Work out the finished part from the listing and answer in its coordinate system (mm). Face numbers are marked on the shaded views. A direction names the side the tool comes from. Round coordinates to 2 decimals unless told otherwise and drop trailing zeros. One line per item, written item: value.
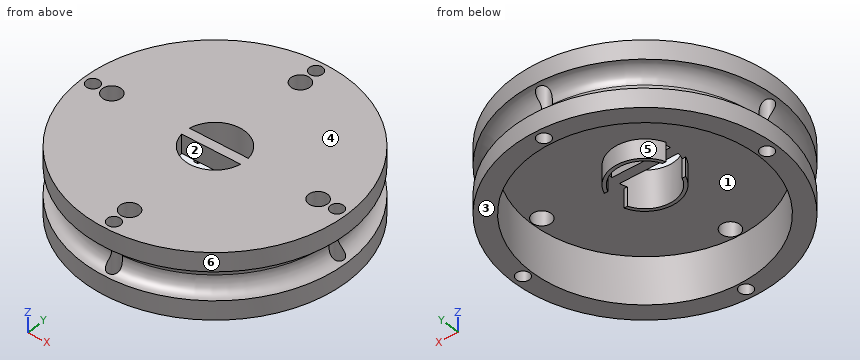
```python
from build123d import *

# Parameters (mm, degrees)
SKETCH1_R               = 14
BOSS_EXTRUDE1_DEPTH     = 7
SKETCH3_R               = 3.15
CUT_EXTRUDE1_DEPTH      = 22
SKETCH4_W               = 7
SKETCH4_H               = 1
BOSS_EXTRUDE2_DEPTH     = 2
SKETCH5_R               = 12
SKETCH5_R_2             = 3.5
CUT_EXTRUDE2_DEPTH      = 5
SKETCH6_W               = 7
SKETCH6_H               = 2.5
CUT_EXTRUDE3_DEPTH      = 5
SKETCH7_R               = 14
SKETCH7_R_2             = 12.5
CUT_EXTRUDE4_DEPTH      = 5
SKETCH8_R               = 14
SKETCH8_R_2             = 12.5
BOSS_EXTRUDE3_DEPTH     = 2
FILLET1_R               = 1.5
CUT_EXTRUDE7_DEPTH      = 22
CUT_EXTRUDE7_DEPTH_BACK = 22
SKETCH9_R               = 1
SKETCH9_R_2             = 0.7
SKETCH10_W              = 6.874413596
SKETCH10_H              = 7.54594332
CUT_EXTRUDE8_DEPTH      = 3


with BuildPart() as part:
    # Sketch1 → Boss-Extrude1 (new body)
    with BuildSketch(Plane.XY):
        Circle(SKETCH1_R)
    extrude(amount=BOSS_EXTRUDE1_DEPTH)

    # Sketch3 → Cut-Extrude1 (cut, through all)
    with BuildSketch(Plane(origin=(0, 0, 0), x_dir=(-1, 0, 0), z_dir=(0, 0, -1))):
        Circle(SKETCH3_R)
    extrude(amount=-CUT_EXTRUDE1_DEPTH, mode=Mode.SUBTRACT)

    # Sketch4 → Boss-Extrude2 (add)
    with BuildSketch(Plane.XY.offset(7)):
        Rectangle(SKETCH4_W, SKETCH4_H)
    extrude(amount=-BOSS_EXTRUDE2_DEPTH)

    # Sketch5 → Cut-Extrude2 (cut)
    with BuildSketch(Plane(origin=(0, 0, 0), x_dir=(-1, 0, 0), z_dir=(0, 0, -1))):
        Circle(SKETCH5_R)
        Circle(SKETCH5_R_2, mode=Mode.SUBTRACT)
    extrude(amount=-CUT_EXTRUDE2_DEPTH, mode=Mode.SUBTRACT)

    # Sketch6 → Cut-Extrude3 (cut)
    with BuildSketch(Plane(origin=(0, 0, 0), x_dir=(-1, 0, 0), z_dir=(0, 0, -1))):
        Rectangle(SKETCH6_W, SKETCH6_H)
    extrude(amount=-CUT_EXTRUDE3_DEPTH, mode=Mode.SUBTRACT)

    # Sketch7 → Cut-Extrude4 (cut)
    with BuildSketch(Plane(origin=(0, 0, 0), x_dir=(-1, 0, 0), z_dir=(0, 0, -1))):
        Circle(SKETCH7_R)
        Circle(SKETCH7_R_2, mode=Mode.SUBTRACT)
    extrude(amount=-CUT_EXTRUDE4_DEPTH, mode=Mode.SUBTRACT)

    # Sketch8 → Boss-Extrude3 (add)
    with BuildSketch(Plane.XY):
        with Locations(Location((0, 0, 0), (0, 0, 180))):
            Circle(SKETCH8_R)
        with Locations(Location((0, 0, 0), (0, 0, 180))):
            Circle(SKETCH8_R_2, mode=Mode.SUBTRACT)
    extrude(amount=BOSS_EXTRUDE3_DEPTH)

    # Fillet1
    fillet1_edges = [part.edges().sort_by_distance(p)[0] for p in [
        (12.5, 0, 5),
        (12.5, 0, 2),
    ]]
    fillet(fillet1_edges, radius=FILLET1_R - 0.0001)  # a hair under: the kernel refuses the full size

    # Sketch9 → Cut-Extrude7 (cut, two sides: drawn at the far end of the back side and taken through both)
    with BuildSketch(Plane(origin=(0, 0, 0), x_dir=(-1, 0, 0), z_dir=(0, 0, -1)).offset(-CUT_EXTRUDE7_DEPTH_BACK)):
        with Locations((0, 10.9)):
            Circle(SKETCH9_R)
        with Locations((0, 12.9)):
            Circle(SKETCH9_R_2)
        with Locations((12.9, 0)):
            Circle(SKETCH9_R_2)
        with Locations((0, -12.9)):
            Circle(SKETCH9_R_2)
        with Locations((-12.9, 0)):
            Circle(SKETCH9_R_2)
        with Locations((-10.9, 0)):
            Circle(SKETCH9_R)
        with Locations((10.9, 0)):
            Circle(SKETCH9_R)
        with Locations((0, -10.9)):
            Circle(SKETCH9_R)
    extrude(amount=CUT_EXTRUDE7_DEPTH + CUT_EXTRUDE7_DEPTH_BACK, mode=Mode.SUBTRACT)

    # Sketch10 → Cut-Extrude8 (cut)
    with BuildSketch(Plane(origin=(0, 0, 0), x_dir=(-1, 0, 0), z_dir=(0, 0, -1))):
        with Locations((0.008465514, -0.14973146)):
            Rectangle(SKETCH10_W, SKETCH10_H)
    extrude(amount=-CUT_EXTRUDE8_DEPTH, mode=Mode.SUBTRACT)


solid = part.part
```
(1) For a pull along Y with two mould halves and no side action, classify the marked faces 4, 5 and 6 as pulls with the +Y half, pulls with the -Y half, needs draft (parallel to the pull), parting line crosses it, or undercut.
Reported:
face 4: needs draft
face 5: undercut
face 6: parting line crosses it
(2) A tool of negligible diameter and unlimited length cuts with its end or side. For the marked faces 1, 2 and 3, from which of +Z, -Z, +X, -X, +Y, -Y can it reach the whole face along a straight path? Write none if from no direction.
Reported:
face 1: -Z
face 2: +Z, -Z
face 3: -Z, +X, -X, +Y, -Y
(3) Consider probe 1 along Y at (x, z) = (0, 3.4); probe 2 along Z at (x, y) = (-3.5, 1.5); probe 3 along Y at (x, z) = (12.9, 1.75). Determine where each line is inside the solid, lowest interval first.
Reported:
probe 1: y = -12.2 to -12, -3.5 to -3.15, 3.15 to 3.5, 12 to 12.2
probe 2: z = 5 to 7
probe 3: y = -5.44 to -0.7, 0.7 to 5.44
(4) Flat-ended cylindrical pins translate along their axes: pin 1 Ø2 at (x, y) = (4, 5.5) entering from -Z; pin 2 Ø1.5 at (y, z) = (-1, 2) entering from -X; pin 3 Ø1.8 at (x, y) = (-0.5, -2.5) entering from -Z; pin 4 Ø1.1 at (x, y) = (0, -12.9) entering from -Z. Find the tip coordinate at first contact, or state that the pin passes through.
Reported:
pin 1: stops at z = 5
pin 2: stops at x = -14
pin 3: stops at z = 3
pin 4: passes through
(5) Find section A-A on z = 5.5. Give the number of separate pieces and of enclosed holes in the cut face, plus the area to 3 significant figures.
Reported:
separate pieces: 1
enclosed holes: 10
area: 572 mm2
